Build history of the part. All positions in model axes, mm. A direction names the side the tool comes from. Round coordinates to 2 decimals unless told otherwise and drop trailing zeros. Write each loop counter-clockwise with the first axis right and the second up, starting at its lowest first coordinate (ties: lowest second). Pieces come first, ordered by that corner, then holes.
Item 1: Drop flat-ended pins along their axis: pin 1 Ø19.5 at (y, z) = (29.5, -2) entering from -X; pin 2 Ø3.5 at (x, z) = (-61, 24.5) entering from -Y. Give the stop position or say it passes through.
Item 2: Wall check: probe 1 along Z at (x, y) = (25.4, 30.5); probe 2 along Z at (x, y) = (25, 11); probe 3 along Z at (x, y) = (22, 20.5). Give the ranges that are in metal, low to high.
Item 3: Band-saw the part on D-D, the plane x = -50.8. Write the cut outline in (y, z) (3 decimals).
Item 4: Band-saw the part on A-A, the plane y = 17.5. Count the separate pieces of the cut face and the enclosed holes in it, then the cut area to 3 significant figures.
Item 5: Mould opens along Z. For faces 4 (the flat face through (-2, 19, 44.45)), 5 (the cylindrical face through (103.865, 18.783, -36.922)), 6 (the flat face through (127, 23, 1)) say: +Z half, -Z half, draft (parallel to the pull), parting line (faces both ways), or undercut.
Item 6: Band-saw the part on B-B, the plane x = 101.6. Write the cut outline in (y, z) (3 decimals), then the cut area to 3 significant figures.
Item 7: Band-saw the part on C-C, the plane x = -11. Write the cut outline in (y, z) (3 decimals), then the cut area to 3 significant figures.
Item 8: 3-axis set-ups, long thin cutter, end or side, ignore diameter. For faces 1 (the flat face through (-2, 16, -19.685)), 2 (the flat face through (-127, 23, 32)), 3 (the flat face through (-24, 29, -13.97)): which of +Z, -Z, +X, -X, +Y, -Y reach the whole face in a straight line?
Autodesk Inventor part; units mm, degrees
ref_plane "YZ Plane" through (0, 0, 0) normal (1, 0, 0) x (0, 1, 0)
ref_plane "XZ Plane" through (0, 0, 0) normal (0, 1, 0) x (-1, 0, 0)
sketch "Sketch1" plane through (0, 0, 0) normal (0, 1, 0) x (-1, 0, 0)
  line L0 (127, 44.45) -> (-127, 44.45)
  line L1 (-127, 44.45) -> (-127, -44.45)
  line L2 (-127, -44.45) -> (127, -44.45)
  line L3 (127, -44.45) -> (127, 44.45)
  line L4 (127, 44.45) -> (-127, -44.45) construction
  line L5 (-127, 44.45) -> (127, -44.45) construction
  point P0 (0, 0)
  dimension "d0" = 254
  dimension "d1" = 88.9
extrude "Extrusion1" add sketch "Sketch1" along normal blind 38.1
sketch "Sketch2" plane through (0, 0, 0) normal (0, -1, 0) x (1, 0, 0)
  line L0 (-131.2333, 19.685) -> (-131.2333, -19.685)
  line L1 (-131.2333, -19.685) -> (131.2333, -19.685)
  line L2 (131.2333, -19.685) -> (131.2333, 19.685)
  line L3 (131.2333, 19.685) -> (-131.2333, 19.685)
  line L4 (-131.2333, 19.685) -> (131.2333, -19.685) construction
  line L5 (-131.2333, -19.685) -> (131.2333, 19.685) construction
  point P0 (0, 0)
  dimension "d4" = 39.37
extrude "Extrusion2" cut sketch "Sketch2" against normal blind 20.32
sketch "Sketch3" plane through (0, 20.32, 0) normal (0, -1, 0) x (1, 0, 0)
  line L0 (-127, -19.685) -> (-127, 19.685)
  line L1 (76.2, 13.97) -> (76.2, -13.97)
  line L2 (76.2, -13.97) -> (-127, -13.97)
  line L3 (-127, -13.97) -> (-127, 13.97)
  line L4 (-127, 13.97) -> (76.2, 13.97)
  line L5 (76.2, 13.97) -> (-127, -13.97) construction
  line L6 (76.2, -13.97) -> (-127, 13.97) construction
  point P0 (0, 0)
  point P1 (-25.4, 0)
  point P2 (-127, -13.97)
  dimension "d7" = 101.6
  dimension "d8" = 27.94
extrude "Extrusion3" cut sketch "Sketch3" against normal through all
sketch "Sketch4" plane through (0, 0, 0) normal (0, -1, 0) x (1, 0, 0)
  line L0 (127, 31.75) -> (-127, 31.75)
  line L1 (-127, 31.75) -> (-127, -31.75)
  line L2 (-127, -31.75) -> (127, -31.75)
  line L3 (127, -31.75) -> (127, 31.75)
  line L4 (127, 31.75) -> (-127, -31.75) construction
  line L5 (-127, 31.75) -> (127, -31.75) construction
  point P0 (0, 0)
  dimension "d11" = 63.5
  dimension "d12" = 254
extrude "Extrusion4" cut sketch "Sketch4" against normal blind 11.43
sketch "Sketch5" plane through (0, 38.1, 0) normal (0, 1, 0) x (1, 0, 0)
  line L0 (127, 44.45) -> (-127, 44.45)
  line L1 (-127, 44.45) -> (-127, 13.97)
  line L2 (-101.6, 38.1) -> (127, 38.1) construction
  line L3 (-101.6, 38.1) -> (-101.6, -44.45) construction
  line L4 (-127, -44.45) -> (127, -44.45) construction
  point P0 (0, 0)
  point P1 (-76.2, 38.1)
  point P2 (-50.8, 38.1)
  point P3 (-25.4, 38.1)
  point P4 (0, 38.1)
  point P5 (25.4, 38.1)
  point P6 (50.8, 38.1)
  point P7 (76.2, 38.1)
  point P8 (101.6, 38.1)
  point P9 (-101.6, -38.1)
  point P10 (-76.2, -38.1)
  point P11 (-50.8, -38.1)
  point P12 (-25.4, -38.1)
  point P13 (0, -38.1)
  point P14 (25.4, -38.1)
  point P15 (50.8, -38.1)
  point P16 (76.2, -38.1)
  point P17 (101.6, -38.1)
  dimension "d15" = 6.35
  dimension "d16" = 25.4
  dimension "d19" = 25.4
  dimension "d22" = 76.2
hole "Hole1" at (-101.6, 38.1, -38.1) at (-76.2, 38.1, -38.1) at (-50.8, 38.1, -38.1) at (-25.4, 38.1, -38.1) at (0, 38.1, -38.1) at (25.4, 38.1, -38.1) at (50.8, 38.1, -38.1) at (76.2, 38.1, -38.1) at (101.6, 38.1, -38.1) at (-101.6, 38.1, 38.1) at (-76.2, 38.1, 38.1) at (-50.8, 38.1, 38.1) at (-25.4, 38.1, 38.1) at (0, 38.1, 38.1) at (25.4, 38.1, 38.1) at (50.8, 38.1, 38.1) at (76.2, 38.1, 38.1) at (101.6, 38.1, 38.1) direction (0, -1, 0) diameter 5.1054 end through all
properties part number "pistonHousingV03-8-in" material "PET Plastic"
Results:
1. pin 1: stops at x = 76.2
1. pin 2: stops at y = 11.43
2. probe 1: z = -44.45 to -40.65, -35.55 to -13.97, 13.97 to 35.55, 40.65 to 44.45
2. probe 2: z = -44.45 to -40.62, -35.58 to -31.75, 31.75 to 35.58, 40.62 to 44.45
2. probe 3: z = -44.45 to -13.97, 13.97 to 44.45
3. outline: (0, -44.45) - (38.1, -44.45) - (38.1, -40.653) - (0, -40.653) - close; (0, -35.547) - (38.1, -35.547) - (38.1, -13.97) - (20.32, -13.97) - (20.32, -19.685) - (11.43, -19.685) - (11.43, -31.75) - (0, -31.75) - close; (0, 31.75) - (11.43, 31.75) - (11.43, 19.685) - (20.32, 19.685) - (20.32, 13.97) - (38.1, 13.97) - (38.1, 35.547) - (0, 35.547) - close; (0, 40.653) - (38.1, 40.653) - (38.1, 44.45) - (0, 44.45) - close
4. separate pieces: 2
4. enclosed holes: 18
4. area: 12,200 mm2
5. face 4: +Z half
5. face 5: undercut
5. face 6: draft
6. outline: (0, -44.45) - (38.1, -44.45) - (38.1, -40.653) - (0, -40.653) - close; (0, -35.547) - (38.1, -35.547) - (38.1, 35.547) - (0, 35.547) - (0, 31.75) - (11.43, 31.75) - (11.43, 19.685) - (20.32, 19.685) - (20.32, -19.685) - (11.43, -19.685) - (11.43, -31.75) - (0, -31.75) - close; (0, 40.653) - (38.1, 40.653) - (38.1, 44.45) - (0, 44.45) - close
6. area: 1,920 mm2
7. outline: (0, -44.45) - (38.1, -44.45) - (38.1, -13.97) - (20.32, -13.97) - (20.32, -19.685) - (11.43, -19.685) - (11.43, -31.75) - (0, -31.75) - close; (0, 31.75) - (11.43, 31.75) - (11.43, 19.685) - (20.32, 19.685) - (20.32, 13.97) - (38.1, 13.97) - (38.1, 44.45) - (0, 44.45) - close
7. area: 1,810 mm2
8. face 1: +X, -X, -Y
8. face 2: +Z, -Z, -X, +Y, -Y
8. face 3: -X, +Y, -Y
